Can you work these out from the model? Positions are in its coordinate system, mm. Face numbers are marked on the shaded views. A direction names the side the tool comes from. Give positions to 0.01 mm unless a question says otherwise; leave off trailing zeros. Loops run counter-clockwise (first coordinate to the right, second up) from the corner with the lowest first, then second, coordinate; pieces in that order, holes last. Notation, with made-up numbers: (-37, -33.75) - (5, -33.75) arc R28 cw to (5, 2.25) - close; hole circle Ø5 at (-7.75, 50.25). An arc over 180 degrees is marked (long way). Write item = value, one per line.
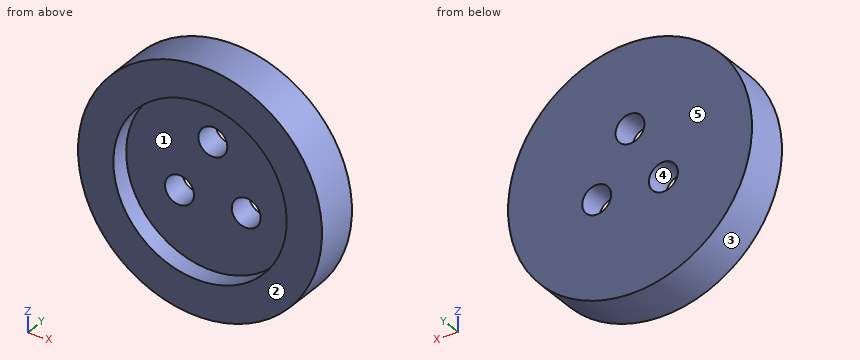
from build123d import *

# Parameters (mm, degrees)
F3_D = 4.5


with BuildPart() as f1:
    # F0 (on Right) → F1 (revolve)
    with BuildSketch(Plane.YZ):
        Polygon((7, 19), (0, 19), (0, 13.5), (3, 13.5), (3, 0), (7, 0), align=None)
    revolve(axis=Axis((0, 5, 0), (0, 1, 0)))

    # F3 (through all)
    with Locations(Plane(origin=(0, 7, 0), x_dir=(-1, 0, 0), z_dir=(0, 1, 0))):
        with Locations((0, 6), (-5.196152, -3), (5.196152, -3)):
            Hole(F3_D / 2)


solid = f1.part
Q1. For pin 1 (13.5 mm diameter, centred on x = -3.5, z = 1, fed in from -Y); pin 2 (1 mm diameter, centred on y = 6, z = 13.5, fed in from -X); pin 3 (1 mm diameter, centred on x = 3.5, y = 3, fed in from -Z), each with a flat end and sliding along its axis, tell me the tip position at first contact or that it passes through.
Output:
pin_1 = 3
pin_2 = -13.86
pin_3 = -18.76
Q2. We'd pull the mould along X, two halves only. Please class the marked faces 3, 4 and 5: released by +X, released by -X, zero draft, split by the parting line, or undercut.
Output:
face_3 = split by the parting line
face_4 = undercut
face_5 = zero draft
Q3. Which directions (+Z, -Z, +X, -X, +Y, -Y) give clear straight access to the entire face, cutting with the end or side of a thin tool? Please do the marked faces 1 and 2.
Output:
face_1 = -Y
face_2 = +Z, -Z, +X, -X, -Y
Q4. Imagine slicing it at D-D, the plane z = 0. Write out the boundary of the cut face in (x, y).
Output:
outline = (-19, 0) - (-13.5, 0) - (-13.5, 3) - (13.5, 3) - (13.5, 0) - (19, 0) - (19, 7) - (-19, 7) - close
Q5. Imagine slicing it at C-C, the plane y = 0.5. Write out the boundary of the cut face in (x, z).
Output:
outline = circle Ø38 at (0, 0); hole circle Ø27 at (0, 0)
Q6. Imagine slicing it at B-B, the plane z = 6. Write out the boundary of the cut face in (x, y).
Output:
outline = (-18.03, 0) - (-12.09, 0) - (-12.09, 3) - (-2.25, 3) - (-2.25, 7) - (-18.03, 7) - close; (2.25, 3) - (12.09, 3) - (12.09, 0) - (18.03, 0) - (18.03, 7) - (2.25, 7) - close
Q7. Imagine slicing it at A-A, the plane x = 0. Write out the boundary of the cut face in (y, z).
Output:
outline = (0, -19) - (7, -19) - (7, 3.75) - (3, 3.75) - (3, -13.5) - (0, -13.5) - close; (0, 13.5) - (3, 13.5) - (3, 8.25) - (7, 8.25) - (7, 19) - (0, 19) - close
Q8. I need wall thicknesses on L1, parallel to X at y = 2.2, z = 0; L2, parallel to X at y = 5.5, z = 0; L3, parallel to Y at x = 0.5, z = 12.5. Which ranges of each line are inside material? Lowest first, please.
Output:
L1 = -19 to -13.5, 13.5 to 19
L2 = -19 to 19
L3 = 3 to 7
